Design review of the part built by this model. Coordinates are the model's own, in mm. A direction names the side the tool comes from. Coordinates: 2 decimals unless noted, no trailing zeros. Loops run counter-clockwise (first coordinate to the right, second up) from the corner with the lowest first, then second, coordinate; pieces in that order, holes last.
Q1. Machinability: for faces 1 (the face through (8.8, 14.8, 9.5)), 2 (the face through (-16, -15, 4.02)), 3 (the face through (30, 8, 15)), 4 (the face through (-17, 5, 19.736)), 5 (the face through (-15, -12, 19.75)), which of the approach directions +Z, -Z, +X, -X, +Y, -Y give a long, thin tool a straight path to every point of the face, cutting with its end or side? Answer none if there is none.
Q2. Draft analysis for pull direction Z (two halves, no side actions). For faces 6 (the face through (-15, -30, 21)), 7 (the face through (-16, -24, 19.457)), state which applies: released by +Z, released by -Z, zero draft, split by the parting line, or undercut.
Q3. Add section C-C on z = 7. Give the boundary of the cut face in (x, y).
Q4. Add section D-D on y = -2.5. Give the boundary of the cut face in (x, z), and give its area (3 significant figures).
Q5. Wall thickness on probe 1 along Z at (x, y) = (-20.5, 13); probe 2 along Z at (x, y) = (-10, -7.5); probe 3 along Y at (x, z) = (21, 18.5): over which ranges is each line inside the solid? List them lowest first.
Q6. Add section B-B on x = 11. Give the boundary of the cut face in (y, z).
Q7. Add section A-A on y = -11. Give the boundary of the cut face in (x, z), and give its area (3 significant figures).
Q8. For P1, Ø4, axis at y = -17, z = 9, coming from the +X side; P2, Ø5, axis at x = -17, z = 13, coming from the +Y side, all flat-tipped, find the tip position at first contact; note any pin that passes through.
```python
from build123d import *

# Parameters (mm, degrees)
F1_DEPTH  = 30
F2_W      = 10
F2_H      = 10
F3_DEPTH  = 30
F4_W      = 10
F4_H      = 10
F5_DEPTH  = 30
F6_W      = 10
F6_H      = 10
F7_DEPTH  = 60
F8_W      = 10
F8_H      = 10
F9_DEPTH  = 60
F10_W     = 10.937084
F10_H     = 15.436338
F11_DEPTH = 30


with BuildPart() as f1:
    # F0 (on Top) → F1 (new body)
    with BuildSketch(Plane.XY):
        Polygon((30, 30), (0, 30), (-30, 30), (-30, 0), (-30, -30), (0, -30), (0, 0), (30, 0), align=None)
    extrude(amount=F1_DEPTH)

    # F2 (on Front) → F3 (cut)
    with BuildSketch(Plane.XZ):
        with Locations((13.8, 14.042104)):
            Rectangle(F2_W, F2_H)
    extrude(amount=-F3_DEPTH, mode=Mode.SUBTRACT)

    # F4 (on face) → F5 (cut)
    with BuildSketch(Plane.YZ):
        with Locations((-12.199999, 14.75)):
            Rectangle(F4_W, F4_H)
    extrude(amount=-F5_DEPTH, mode=Mode.SUBTRACT)

    # F6 (on face) → F7 (cut)
    with BuildSketch(Plane(origin=(-30, 0, 0), x_dir=(0, -1, 0), z_dir=(-1, 0, 0))):
        with Locations((-14.900001, 14.75)):
            Rectangle(F6_W, F6_H)
    extrude(amount=-F7_DEPTH, mode=Mode.SUBTRACT)

    # F8 (on Front) → F9 (cut)
    with BuildSketch(Plane.XZ):
        with Locations((-16.978183, 14.736477)):
            Rectangle(F8_W, F8_H)
    extrude(amount=-F9_DEPTH, mode=Mode.SUBTRACT)

    # F10 (on face) → F11 (cut)
    with BuildSketch(Plane.XZ.offset(30)):
        with Locations((-15.822794, 11.738348)):
            Rectangle(F10_W, F10_H)
    extrude(amount=-F11_DEPTH, mode=Mode.SUBTRACT)


with BuildPart() as f12_1:
    # F12: copy of F1
    add(f1.part)


solid = f1.part
```
Entries:
1. face 1: +Y, -Y
1. face 2: -Y
1. face 3: +Z, -Z, +X, +Y, -Y
1. face 4: +Y
1. face 5: +X, -X
2. face 6: zero draft
2. face 7: undercut
3. outline: (-30, -30) - (-21.29, -30) - (-21.29, 0) - (-10.35, 0) - (-10.35, -30) - (0, -30) - (0, 0) - (30, 0) - (30, 30) - (-30, 30) - close
4. outline: (-30, 0) - (0, 0) - (0, 30) - (-30, 30) - close; hole (-21.29, 4.02) - (-10.35, 4.02) - (-10.35, 19.46) - (-21.29, 19.46) - close
4. area: 731 mm2
5. probe 1: z = 0 to 9.74, 19.75 to 30
5. probe 2: z = 0 to 9.75, 19.75 to 30
5. probe 3: y = 0 to 9.9, 19.9 to 30
6. outline: (0, 0) - (30, 0) - (30, 9.04) - (0, 9.04) - close; (0, 19.04) - (9.9, 19.04) - (9.9, 19.75) - (19.9, 19.75) - (19.9, 19.04) - (30, 19.04) - (30, 30) - (0, 30) - close
7. outline: (-30, 0) - (0, 0) - (0, 9.75) - (-10.35, 9.75) - (-10.35, 4.02) - (-21.29, 4.02) - (-21.29, 9.75) - (-30, 9.75) - close; (-30, 19.75) - (0, 19.75) - (0, 30) - (-30, 30) - close
7. area: 537 mm2
8. P1: stops at x = 0
8. P2: passes through
